Check sheet for the modelled part. Datum: model origin and axes. Units: mm. A direction names the side the tool comes from. Coordinates: 2 decimals unless noted, no trailing zeros. Loops run counter-clockwise (first coordinate to the right, second up) from the corner with the lowest first, then second, coordinate; pieces in that order, holes last. Notation, with made-up numbers: (48.25, 1) -> (88.25, 1) arc R29 cw to (88.25, 22) -> close; hole circle Ø11 at (65, -29). An arc over 180 degrees is marked (long way). Use CSV: the item, a comma, the result in double quotes.
```python
from build123d import *

# Parameters (mm, degrees)
F0_W     = 241.3
F0_H     = 120.65
F1_DEPTH = 9.525
F2_R     = 12.7
F3_R     = 38.1
F5_D     = 12.7
F6_R     = 25.4
F8_D     = 7.9375
F10_D    = 7.9375
F12_D    = 7.9375


# Not quite as in the source:
# - a length typed as a fraction of an inch, garbled in the dataset ("3 / 203.2 mm" for 3/8 in), is restored


with BuildPart() as f1:
    # F0 (on Front) → F1 (new body, symmetric)
    with BuildSketch(Plane.XZ):
        Polygon((-38.1, 0), (0, 0), (0, 374.65), (-432.054, 374.65), (-432.054, 457.2), (-470.154, 457.2), (-470.154, 336.55), (-317.5, 336.55), (-317.5, 0), (-279.4, 0), (-279.4, 177.8), (-38.1, 177.8), align=None)
        with Locations((-158.75, 276.225)):
            Rectangle(F0_W, F0_H, mode=Mode.SUBTRACT)
    extrude(amount=F1_DEPTH, both=True)

    # F2
    f2_edges = [f1.edges().sort_by_distance(p)[0] for p in [
        (-279.4, 0, 336.55),
        (-279.4, 0, 215.9),
        (-38.1, 0, 215.9),
        (-38.1, 0, 336.55),
        (-279.4, 0, 177.8),
        (-38.1, 0, 177.8),
    ]]
    fillet(f2_edges, radius=F2_R)

    # F3
    f3_edges = [f1.edges().sort_by_distance(p)[0] for p in [
        (-317.5, 0, 336.55),
        (-432.054, 0, 374.65),
    ]]
    fillet(f3_edges, radius=F3_R)

    # F5 (through all)
    with Locations(Plane.YZ):
        with Locations((0, 9.525)):
            Hole(F5_D / 2)

    # F6
    f6_edges = [f1.edges().sort_by_distance(p)[0] for p in [
        (-470.154, 0, 336.55),
        (0, 0, 374.65),
    ]]
    fillet(f6_edges, radius=F6_R)

    # F8 (through all)
    with Locations(Plane.XZ.offset(9.525)):
        with Locations((-174.625, 355.6), (-142.875, 355.6)):
            Hole(F8_D / 2)

    # F10 (through all)
    with Locations(Plane(origin=(0, 9.525, 0), x_dir=(-1, 0, 0), z_dir=(0, 1, 0))):
        with Locations((9.525, 320.675), (9.525, 339.725)):
            Hole(F10_D / 2)

    # F12 (through all)
    with Locations(Plane.XZ.offset(9.525)):
        with Locations((-457.454, 415.925), (-457.454, 396.875)):
            Hole(F12_D / 2)


solid = f1.part
```
1) Access from +Z, -Z, +X, -X, +Y, -Y to the whole of each face (thin tool, end or side, straight path). Record for faces 4 (the flat face through (-317.5, 0, 151)), 5 (the flat face through (-160, 0, 215.9)), 6 (the flat face through (-279.4, 0, 81)), 7 (the flat face through (-207, 0, 374.65)).
Answer below:
face 4,"-Z, -X, +Y, -Y"
face 5,"+Y, -Y"
face 6,"-Z, +Y, -Y"
face 7,"+Z, +X, +Y, -Y"
2) Cross-section at A-A on x = -114. Record the boundary of the cut face in (y, z) (3 decimals), and give its area (3 significant figures).
Answer below:
outline,"(-9.525, 177.8) -> (9.525, 177.8) -> (9.525, 215.9) -> (-9.525, 215.9) -> close; (-9.525, 336.55) -> (9.525, 336.55) -> (9.525, 374.65) -> (-9.525, 374.65) -> close"
area,"1,450 mm²"
3) Thickness scan on line 1 along X through (y, z) = (-2.5, 272); line 2 along Z through (x, y) = (-117.5, -7.5); line 3 along X through (y, z) = (-5.75, 356). Record the ranges inside material, lowest first. Write a range as from..to.
Answer below:
line 1,"x = -317.5..-279.4, -38.1..0"
line 2,"z = 177.8..215.9, 336.55..374.65"
line 3,"x = -469.45..-178.57, -170.68..-146.82, -138.93..-0.91"
4) Cross-section at C-C on y = 1.25. Give the number of separate pieces and of enclosed holes in the cut face, and give its area (3 significant figures).
Answer below:
separate pieces,"3"
enclosed holes,"7"
area,"55,200 mm²"
5) Go/stop test with flat-tipped pins: pin 1 Ø5.5 at (y, z) = (2, 260) entering from -X; pin 2 Ø1 at (x, y) = (-155, -6) entering from -Z; pin 3 Ø1 at (y, z) = (4.5, 385) entering from +X. Record where each tip stops, or that it passes through.
Answer below:
pin 1,"stops at x = -317.5"
pin 2,"stops at z = 177.8"
pin 3,"stops at x = -419.52"
6) Draft check along Z on faces 1 (the cylindrical face through (-41.72, 0.13, 173.98)), 2 (the flat face through (-201, 9.525, 213)), 3 (the cylindrical face through (-275.78, 0.13, 332.73)). Enter one of: released by +Z, released by -Z, zero draft, split by the parting line, or undercut.
Answer below:
face 1,"released by -Z"
face 2,"zero draft"
face 3,"undercut"
7) Cross-section at B-B on z = 253.5. Record the boundary of the cut face in (x, y) (3 decimals), and give its area (3 significant figures).
Answer below:
outline,"(-317.5, -9.525) -> (-279.4, -9.525) -> (-279.4, 9.525) -> (-317.5, 9.525) -> close; (-38.1, -9.525) -> (0, -9.525) -> (0, 9.525) -> (-38.1, 9.525) -> close"
area,"1,450 mm²"
